```python
from build123d import *

# Parameters (mm, degrees)
EXTRUDE_START            = 5
EXTRUDE_3_Z5_DEPTH       = 3
CUT_EXTRUDE_START        = 5
CUT_EXTRUDE_U_18_DEPTH   = 3
EXTRUDE_START_2          = 3
SKETCH_3_R               = 2.75
EXTRUDE_2_Z3_5_DEPTH     = 2
SKETCH_4_R               = 2
EXTRUDE_3_Z0_3_DEPTH     = 3
SKETCH_5_R               = 1.1
CUT_EXTRUDE_2X_2_2_DEPTH = 8
CUT_EXTRUDE_START_2      = 5.9
SKETCH_6_R               = 2.1
CUT_EXTRUDE_2_1_DEPTH    = 2.1
SKETCH_7_R               = 1.8
CUT_EXTRUDE_4X_3_6_DEPTH = 3


with BuildPart() as part:
    # 草图1 → 背板拉伸_厚3_前面Z5 (new body)
    with BuildSketch(Plane.XY.offset(EXTRUDE_START)):
        with BuildLine():
            Line((-16, -13), (16, -13))
            ThreePointArc((16, -13), (17.414213562, -12.414213562), (18, -11))
            Line((18, -11), (18, 11))
            ThreePointArc((18, 11), (17.414213562, 12.414213562), (16, 13))
            Line((16, 13), (-16, 13))
            ThreePointArc((-16, 13), (-17.414213562, 12.414213562), (-18, 11))
            Line((-18, 11), (-18, -11))
            ThreePointArc((-18, -11), (-17.414213562, -12.414213562), (-16, -13))
        make_face()
    extrude(amount=EXTRUDE_3_Z5_DEPTH)

    # 草图2 → 下方U口_宽18_向下敞开 (cut)
    with BuildSketch(Plane.XY.offset(CUT_EXTRUDE_START)):
        with BuildLine():
            Line((-8, -20), (8, -20))
            ThreePointArc((8, -20), (8.707106781, -19.707106781), (9, -19))
            Line((9, -19), (9, -4.5))
            ThreePointArc((9, -4.5), (8.707106781, -3.792893219), (8, -3.5))
            Line((8, -3.5), (-8, -3.5))
            ThreePointArc((-8, -3.5), (-8.707106781, -3.792893219), (-9, -4.5))
            Line((-9, -4.5), (-9, -19))
            ThreePointArc((-9, -19), (-8.707106781, -19.707106781), (-8, -20))
        make_face()
    extrude(amount=CUT_EXTRUDE_U_18_DEPTH, mode=Mode.SUBTRACT)

    # 草图3 → 两根支柱主体_高2_Z3至5 (add)
    with BuildSketch(Plane.XY.offset(EXTRUDE_START_2)):
        with Locations((-7.2, 0)):
            Circle(SKETCH_3_R)
        with Locations((7.2, 0)):
            Circle(SKETCH_3_R)
    extrude(amount=EXTRUDE_2_Z3_5_DEPTH)

    # 草图4 → 两根接触细颈_高3_Z0至3 (add)
    with BuildSketch(Plane.XY):
        with Locations((-7.2, 0)):
            Circle(SKETCH_4_R)
        with Locations((7.2, 0)):
            Circle(SKETCH_4_R)
    extrude(amount=EXTRUDE_3_Z0_3_DEPTH)

    # 草图5 → 模块固定孔_2x直径2.2_贯穿 (cut)
    with BuildSketch(Plane.XY):
        with Locations((-7.2, 0)):
            Circle(SKETCH_5_R)
        with Locations((7.2, 0)):
            Circle(SKETCH_5_R)
    extrude(amount=CUT_EXTRUDE_2X_2_2_DEPTH, mode=Mode.SUBTRACT)

    # 草图6 → 背面螺丝头沉孔_深2.1 (cut)
    with BuildSketch(Plane.XY.offset(CUT_EXTRUDE_START_2)):
        with Locations((-7.2, 0)):
            Circle(SKETCH_6_R)
        with Locations((7.2, 0)):
            Circle(SKETCH_6_R)
    extrude(amount=CUT_EXTRUDE_2_1_DEPTH, mode=Mode.SUBTRACT)

    # 草图7 → 后续连接孔_4x直径3.6_贯穿 (cut)
    with BuildSketch(Plane.XY.offset(CUT_EXTRUDE_START)):
        with Locations((-13.5, -9)):
            Circle(SKETCH_7_R)
        with Locations((-13.5, 9)):
            Circle(SKETCH_7_R)
        with Locations((13.5, -9)):
            Circle(SKETCH_7_R)
        with Locations((13.5, 9)):
            Circle(SKETCH_7_R)
    extrude(amount=CUT_EXTRUDE_4X_3_6_DEPTH, mode=Mode.SUBTRACT)


solid = part.part
```
Part model, mm, in its own coordinate system. A direction names the side the tool comes from. Round coordinates to 2 decimals unless told otherwise and drop trailing zeros. Write each loop counter-clockwise with the first axis right and the second up, starting at its lowest first coordinate (ties: lowest second). Pieces come first, ordered by that corner, then holes. Notation, with made-up numbers: (75.5, 7) -> (87.5, 7) arc R16 cw to (87.5, 19) -> close; hole circle Ø1 at (62.25, -12). An arc over 180 degrees is marked (long way). Return JSON: item names as keys, results as strings. Group by question number.
Q1. Mould opens along Y. For faces 1 (the cylindrical face through (6.1, 0, 2.9)), 2 (the flat face through (0, -3.5, 6)), 3 (the flat face through (-9, -9, 6)) say: pulls with the +Y half, pulls with the -Y half, needs draft (parallel to the pull), parting line crosses it, or undercut.
Q2. Saw through at B-B on x = 13.5. Write the cut outline in (y, z).
Q3. Probe L1, parallel to Y at x = -7.2, z = 1.6; L2, parallel to Y at x = 7.2, z = 4.3; L3, parallel to Z at x = 1.5, y = 7.75. List the from-to ranges inside material, lowest first. Write a range as [from, to].
Q4. Which spindle directions (+Z, -Z, +X, -X, +Y, -Y) get a long thin tool onto all of the face, cutting with end or side? Do faces 4 (the cylindrical face through (9.203, 0.631, 6.935)), 5 (the flat face through (9, -9, 6)), 6 (the cylindrical face through (6.766, -1.952, 1.479)), 7 (the flat face through (-18, 0, 6)), 8 (the flat face through (12, -13, 6)). Say none if no direction does.
Q5. Saw through at A-A on y = 9. Write the cut outline in (x, z), plus the area to 3 significant figures.
Q6. Saw through at D-D on z = 1.5. Write the cut outline in (x, y).
Q7. Saw through at C-C on y = -9. Write the cut outline in (x, z).
Q8. Pin check, flat tips, straight feed: pin 1 (1.8 mm diameter, centred on x = -7.2, y = 0, fed in from -Z); pin 2 (6 mm diameter, centred on x = 8, y = -1.5, fed in from -Z); pin 3 (2 mm diameter, centred on x = 9.5, z = 1, fed in from +Y); pin 4 (8 mm diameter, centred on x = 1.5, y = -6, fed in from -Z). Stop position of each tip, or through.
Answer:
{
 "1": {"face 1": "undercut", "face 2": "pulls with the -Y half", "face 3": "needs draft"},
 "2": {"outline": "(-13, 5) -> (-10.8, 5) -> (-10.8, 8) -> (-13, 8) -> close; (-7.2, 5) -> (7.2, 5) -> (7.2, 8) -> (-7.2, 8) -> close; (10.8, 5) -> (13, 5) -> (13, 8) -> (10.8, 8) -> close"},
 "3": {"L1": "[-2, -1.1], [1.1, 2]", "L2": "[-2.75, -1.1], [1.1, 2.75]", "L3": "[5, 8]"},
 "4": {"face 4": "+Z", "face 5": "+Z, -Z, -Y", "face 6": "-Z", "face 7": "+Z, -Z, -X, +Y, -Y", "face 8": "+Z, -Z, +X, -X, -Y"},
 "5": {"outline": "(-18, 5) -> (-15.3, 5) -> (-15.3, 8) -> (-18, 8) -> close; (-11.7, 5) -> (11.7, 5) -> (11.7, 8) -> (-11.7, 8) -> close; (15.3, 5) -> (18, 5) -> (18, 8) -> (15.3, 8) -> close", "area": "86.4 mm2"},
 "6": {"outline": "circle Ø4 at (-7.2, 0); circle Ø4 at (7.2, 0); hole circle Ø2.2 at (-7.2, 0); hole circle Ø2.2 at (7.2, 0)"},
 "7": {"outline": "(-18, 5) -> (-15.3, 5) -> (-15.3, 8) -> (-18, 8) -> close; (-11.7, 5) -> (-9, 5) -> (-9, 8) -> (-11.7, 8) -> close; (9, 5) -> (11.7, 5) -> (11.7, 8) -> (9, 8) -> close; (15.3, 5) -> (18, 5) -> (18, 8) -> (15.3, 8) -> close"},
 "8": {"pin 1": "through", "pin 2": "z = 0", "pin 3": "y = 1.52", "pin 4": "z = 5"}
}
